```python
from build123d import *

# Parameters (mm, degrees)
EXTRUDE1_DEPTH     = 228.6
CUT_EXTRUDE1_DEPTH = 123.825
CUT_EXTRUDE2_DEPTH = 73.025
CUT_EXTRUDE3_DEPTH = 73.025
SKETCH6_W          = 1.5875
SKETCH6_H          = 19.05
CUT_EXTRUDE4_DEPTH = 184.15


with BuildPart() as part:
    # Sketch2 → Extrude1 (new body, symmetric)
    with BuildSketch(Plane.XY):
        Polygon((101.6, 12.7), (101.6, 0), (139.7, 0), (139.7, 20.6375), (138.1125, 20.6375), (138.1125, 1.5875), (125.449578796, 1.5875), (111.549753001, 65.526698647), (109.998485525, 65.189466588), (123.825, 1.5875), (103.1875, 1.5875), (103.1875, 12.7), align=None)
    extrude(amount=EXTRUDE1_DEPTH, both=True)

    # Sketch3 → Cut-Extrude1 (cut, symmetric)
    with BuildSketch(Plane.XY):
        Polygon((103.1875, 1.5875), (138.1125, 1.5875), (138.1125, 20.6375), (111.549753001, 65.526698647), (109.998485525, 65.189466588), (103.1875, 12.7), align=None)
    extrude(amount=CUT_EXTRUDE1_DEPTH, both=True, mode=Mode.SUBTRACT)

    # Sketch4 → Cut-Extrude2 (cut)
    with BuildSketch(Plane.XY.offset(228.6)):
        Polygon((103.1875, 12.7), (103.1875, 1.5875), (138.1125, 1.5875), (138.1125, 20.6375), (111.549753001, 65.526698647), (109.998485525, 65.189466588), align=None)
    extrude(amount=-CUT_EXTRUDE2_DEPTH, mode=Mode.SUBTRACT)

    # Sketch5 → Cut-Extrude3 (cut)
    with BuildSketch(Plane(origin=(0, 0, -228.6), x_dir=(-1, 0, 0), z_dir=(0, 0, -1))):
        Polygon((-138.1125, 20.6375), (-138.1125, 1.5875), (-103.1875, 1.5875), (-103.1875, 12.7), (-109.998485525, 65.189466588), (-111.549753001, 65.526698647), align=None)
    extrude(amount=-CUT_EXTRUDE3_DEPTH, mode=Mode.SUBTRACT)

    # Sketch6 → Cut-Extrude4 (cut, symmetric)
    with BuildSketch(Plane.XY):
        with Locations((138.90625, 11.1125)):
            Rectangle(SKETCH6_W, SKETCH6_H)
    extrude(amount=CUT_EXTRUDE4_DEPTH, both=True, mode=Mode.SUBTRACT)


solid = part.part
```
Input: part model. Units: mm. Frame: model coordinates. A direction names the side the tool comes from. Give positions to 0.01 mm unless a question says otherwise; leave off trailing zeros. Loops run counter-clockwise (first coordinate to the right, second up) from the corner with the lowest first, then second, coordinate; pieces in that order, holes last. Notation, with made-up numbers: M 27.25,65 L 44.25,65 A24 ccw 44.25,85 Z; hole C 7,43.5 d10. An arc over 180 degrees is marked long. Answer as CSV lines item,"result". Start each with the question number.
1. Pull-direction query (X, two-part tool) for faces 5 (the face through (118, 34, -155.575)), 6 (the face through (122, 1.588, 3)), 7 (the face through (139.7, 0.3, 1.1)); classes: released by +X, released by -X, zero draft, split by the parting line, or undercut.
2. Section B-B on x = 120. Return loops of the section in (y, z) (1 decimal).
3. Section A-A on y = 7. State how many separate pieces and enclosed holes the cut face has, plus the area to 3 significant figures.
4. Line query: L1, parallel to Y at x = 135, z = 82; L2, parallel to X at y = 38, z = -138.5. Output: solid intervals per line, ascending.
5. Pin query (flat end, axial travel): P1, Ø1.7, axis at x = 138.5, z = 204, coming from the +Y side; P2, Ø4, axis at x = 121.5, z = -116, coming from the -Y side; P3, Ø18.5, axis at x = 128, z = 55.5, coming from the +Y side; P4, Ø17, axis at x = 116, y = 29, coming from the -Z side (3 decimals). Return the tip coordinate at first contact, or that it passes through.
6. Section C-C on z = 9.5. Return loops of the section in (x, y), plus the area to 3 significant figures.
7. Reachability of faces 1 (the face through (118, 34, -123.825)), 2 (the face through (116.815, 33.834, -139.478)), 3 (the face through (138.112, 11, 207)), 4 (the face through (118, 34, 155.575)) from +Z, -Z, +X, -X, +Y, -Y: full face, straight path, thin tool, end or side. Return the list, or none.
8. Section D-D on y = 36. Return loops of the section in (x, z) (3 decimals), plus the area to 3 significant figures.
Computed values:
1,face 5,"zero draft"
1,face 6,"undercut"
1,face 7,"released by +X"
2,outline,"M 0,-228.6 L 1.6,-228.6 L 1.6,228.6 L 0,228.6 Z; M 19.2,-155.6 L 26.7,-155.6 L 26.7,-123.8 L 19.2,-123.8 Z; M 19.2,123.8 L 26.7,123.8 L 26.7,155.6 L 19.2,155.6 Z"
3,separate pieces,"5"
3,enclosed holes,"0"
3,area,"970 mm²"
4,L1,"y = 0 to 1.59"
4,L2,"x = 115.91 to 117.53"
5,P1,"stops at y = 20.64"
5,P2,"stops at y = 0"
5,P3,"stops at y = 1.59"
5,P4,"stops at z = -155.575"
6,outline,"M 101.6,0 L 139.7,0 L 139.7,1.59 L 103.19,1.59 L 103.19,12.7 L 101.6,12.7 Z"
6,area,"78.1 mm²"
7,face 1,"+X, +Y"
7,face 2,"+Z, -Z"
7,face 3,"+Z, -Z, +Y"
7,face 4,"+Z, +X, +Y"
8,outline,"M 116.344,-155.575 L 117.969,-155.575 L 117.969,-123.825 L 116.344,-123.825 Z; M 116.344,123.825 L 117.969,123.825 L 117.969,155.575 L 116.344,155.575 Z"
8,area,"103 mm²"
